```python
from build123d import *

# Parameters (mm, degrees)
BOSS_EXTRUDE1_DEPTH      = 725
BOSS_EXTRUDE1_DEPTH_BACK = 725
SKETCH1_R                = 80.75
SKETCH1_R_2              = 78.35
SKETCH2_W                = 5
SKETCH2_H                = 210
CUT_EXTRUDE1_DEPTH       = 734.938774694
CIRPATTERN1_START        = -725
CIRPATTERN1_DEPTH        = 210


# Read off the part's stored shape, not the designer's step: CirPattern1
with BuildPart() as part:
    # Sketch1 → Boss-Extrude1 (new, two sides: drawn at the far end of the back side and taken through both)
    with BuildSketch(Plane(origin=(0, 0, 0), x_dir=(1, 0, 0), z_dir=(0, 1, 0)).offset(-BOSS_EXTRUDE1_DEPTH_BACK)):
        with Locations(Location((0, 0, 0), (0, 0, 270))):
            Circle(SKETCH1_R)
        with Locations(Location((0, 0, 0), (0, 0, 270))):
            Circle(SKETCH1_R_2, mode=Mode.SUBTRACT)
    extrude(amount=BOSS_EXTRUDE1_DEPTH + BOSS_EXTRUDE1_DEPTH_BACK)

    # Sketch2 → Cut-Extrude1 (cut, symmetric)
    with BuildSketch(Plane.XY):
        with Locations((0, -620)):
            Rectangle(SKETCH2_W, SKETCH2_H)
    extrude(amount=CUT_EXTRUDE1_DEPTH, both=True, mode=Mode.SUBTRACT)

    # CirPattern1 outline → CirPattern1 (cut)
    with BuildSketch(Plane(origin=(0, 0, 0), x_dir=(1, 0, 0), z_dir=(0, 1, 0)).offset(CIRPATTERN1_START)):
        with BuildLine():
            ThreePointArc((-80.711291032, 2.5), (-80.75, 0), (-80.711291032, -2.5))
            Line((-80.711291032, -2.5), (-78.310104712, -2.5))
            ThreePointArc((-78.310104712, -2.5), (-78.35, 0), (-78.310104712, 2.5))
            Line((-78.310104712, 2.5), (-80.711291032, 2.5))
        make_face()
        with BuildLine():
            Line((78.310104712, -2.5), (80.711291032, -2.5))
            ThreePointArc((80.711291032, -2.5), (80.75, 0), (80.711291032, 2.5))
            Line((80.711291032, 2.5), (78.310104712, 2.5))
            ThreePointArc((78.310104712, 2.5), (78.35, 0), (78.310104712, -2.5))
        make_face()
    extrude(amount=CIRPATTERN1_DEPTH, mode=Mode.SUBTRACT)


solid = part.part
```
Geometry: final body of the model. Coordinates: model frame, mm. Round coordinates to 2 decimals unless told otherwise and drop trailing zeros. Order: outer loops, then holes, each group sorted by start corner. A loop starts at its lowest first (then second) coordinate and runs counter-clockwise, first axis right, second up. Notation, with made-up numbers: M 74.25,88.25 L 99.25,88.25 A15 ccw 99.25,106.25 Z; hole C -21,77.5 d2. An arc over 180 degrees is marked long. One line per item, written item: value.
(1) Line query: probe 1 along X at (y, z) = (-419, 0); probe 2 along X at (y, z) = (-329.5, -26.5). Output: solid intervals per line, ascending. Write a range as [from, to].
Result sheet:
probe 1: [-80.75, -78.35], [78.35, 80.75]
probe 2: [-76.28, -73.73], [73.73, 76.28]
(2) Cut plane D-D (y = -262). Return the cut outline in (x, z), and give its area (3 significant figures).
Result sheet:
outline: C 0,0 d161.5; hole C 0,0 d156.7
area: 1,200 mm2
(3) Pull-direction query (X, two-part tool) for faces 1 (the cylindrical face through (54.57, -10.15, -59.52)), 2 (the flat face through (-56, -725, -56)), 3 (the cylindrical face through (23.534, -10.15, 74.732)); classes: pulls with the +X half, pulls with the -X half, needs draft (parallel to the pull), parting line crosses it, or undercut.
Result sheet:
face 1: parting line crosses it
face 2: needs draft
face 3: undercut
(4) Cut plane A-A (y = -633). Return the cut outline in (x, z).
Result sheet:
outline: M -80.71,-2.5 A80.75 ccw -2.5,-80.71 L -2.5,-78.31 A78.35 cw -78.31,-2.5 Z; M -80.71,2.5 L -78.31,2.5 A78.35 cw -2.5,78.31 L -2.5,80.71 A80.75 ccw Z; M 2.5,-80.71 A80.75 ccw 80.71,-2.5 L 78.31,-2.5 A78.35 cw 2.5,-78.31 Z; M 2.5,78.31 A78.35 cw 78.31,2.5 L 80.71,2.5 A80.75 ccw 2.5,80.71 Z
(5) Cut plane B-B (x = -56). Return the cut outline in (y, z), and give its area (3 significant figures).
Result sheet:
outline: M -725,-58.18 L 725,-58.18 L 725,-54.8 L -725,-54.8 Z; M -725,54.8 L 725,54.8 L 725,58.18 L -725,58.18 Z
area: 9,800 mm2
(6) Cut plane C-C (z = -35). Return the cut outline in (x, y), and give its area (3 significant figures).
Result sheet:
outline: M -72.77,-725 L -70.1,-725 L -70.1,725 L -72.77,725 Z; M 70.1,-725 L 72.77,-725 L 72.77,725 L 70.1,725 Z
area: 7,750 mm2
(7) Pin query (flat end, axial travel): P1, Ø5, axis at x = 49, y = -355.5, coming from the +Z side; P2, Ø5, axis at x = -58.5, y = -128.5, coming from the -Z side; P3, Ø10, axis at x = 7.5, y = -357.5, coming from the -Z side. Return the tip coordinate at first contact, or that it passes through.
Result sheet:
P1: z = 66.02
P2: z = -58.18
P3: z = -80.71
